CAD build for the part. Positions are in the model's coordinates, mm. A direction names the side the tool comes from. Give positions to 0.01 mm unless a question says otherwise; leave off trailing zeros. Loops run counter-clockwise (first coordinate to the right, second up) from the corner with the lowest first, then second, coordinate; pieces in that order, holes last. Notation, with made-up numbers: M 11,-20.75 L 35,-20.75 A28 ccw 35,3.25 Z; hole C 16.25,15 d8. An arc over 180 degrees is marked long. One line per question, with ' | ' between items.
```python
from build123d import *

# Parameters (mm, degrees)
F1_DEPTH  = 140
F3_DEPTH  = 25
F4_W      = 14.9999646693
F4_H      = 12.7701332697
F4_W_2    = 15
F5_DEPTH  = 2
F6_R      = 2
F7_W      = 11
F7_H      = 12
F8_DEPTH  = 2
F10_DEPTH = 50
F12_D     = 4.4


with BuildPart() as f1:
    # F0 (on Front) → F1 (new body)
    with BuildSketch(Plane.XZ):
        Polygon((-5.5, 12), (-7.5, 12), (-7.5, 0), (7.5, 0), (7.5, 12), (5.5, 12), (5.5, 2), (-5.5, 2), align=None)
    extrude(amount=F1_DEPTH)

    # F2 (on face) → F3 (cut)
    with BuildSketch(Plane(origin=(-7.5, 0, 0), x_dir=(0, -1, 0), z_dir=(-1, 0, 0))):
        Polygon((4.3676428112, 0), (0, 12), (0, 0), align=None)
    extrude(amount=-F3_DEPTH, mode=Mode.SUBTRACT)

    # F4 (on face) → F5 (join)
    with BuildSketch(Plane(origin=(0, -3.8567256581, 1.4037333413), x_dir=(-1, 0, 0), z_dir=(0, 0.9396926208, -0.3420201433))):
        with Locations((-12.9999823347, 4.8912448146)):
            Rectangle(F4_W, F4_H)
        with Locations((13, 4.8912448146)):
            Rectangle(F4_W_2, F4_H)
    extrude(amount=F5_DEPTH)

    # F6
    f6_edges = [f1.edges().sort_by_distance(p)[0] for p in [
        (20.499965, 0.939693, 11.65798),
        (-20.5, 0.939693, 11.65798),
        (20.499965, -3.42795, -0.34202),
        (-20.5, -3.42795, -0.34202),
    ]]
    fillet(f6_edges, radius=F6_R)

    # F7 (on face) → F8 (join)
    with BuildSketch(Plane(origin=(0, 0, 0), x_dir=(1, 0, 0), z_dir=(0, 0, -1))):
        with Locations((0, -1.6323571888)):
            Rectangle(F7_W, F7_H)
    extrude(amount=-F8_DEPTH)

    # F9 (on face) → F10 (cut, symmetric)
    with BuildSketch(Plane(origin=(-5.5, 0, 0), x_dir=(0, -1, 0), z_dir=(-1, 0, 0))):
        Polygon((2.2392872662, 0), (-7.6323571888, 0), (-7.6323571888, -1.849311986), (7.0655047894, -1.849311986), (7.0655047894, 0), align=None)
    extrude(amount=F10_DEPTH, both=True, mode=Mode.SUBTRACT)

    # F12 (through all)
    with Locations(Plane(origin=(0, -1.9773404165, 0.7196930546), x_dir=(-1, 0, 0), z_dir=(0, 0.9396926208, -0.3420201433))):
        with Locations((-12.5, 5.2763114494), (12.5, 5.2763114494)):
            Hole(F12_D / 2)


solid = f1.part
```
Item 1: Drill centre lines: line 1 along X through (y, z) = (-130.5, 11); line 2 along Z through (x, y) = (1, -122.5); line 3 along Y through (x, z) = (-17, 6.5). Where is each one in solid material? Low to high. Write a range as [from, to].
Conclusion:
line 1: [-7.5, -5.5], [5.5, 7.5] | line 2: [0, 2] | line 3: [-2, 0.13]
Item 2: Saw through at B-B on x = -13. Give the cut face in (y, z), and give its area (3 significant figures).
Conclusion:
outline: M -4.37,0 L -2.24,0 L -0.91,3.66 L -2.78,4.35 Z; M -1.32,8.38 L 0.56,7.69 L 1.88,11.32 L 0,12 Z | area: 16.2 mm²
Item 3: Saw through at A-A on y = -66.5. Give the cut face in (x, z), and give its area (3 significant figures).
Conclusion:
outline: M -7.5,0 L 7.5,0 L 7.5,12 L 5.5,12 L 5.5,2 L -5.5,2 L -5.5,12 L -7.5,12 Z | area: 70.0 mm²
Item 4: Saw through at C-C on x = -3.5. Give the cut face in (y, z).
Conclusion:
outline: M -140,0 L 7.63,0 L 7.63,2 L -140,2 Z
Item 5: Saw through at D-D on x = 17. Give the cut face in (y, z), and give its area (3 significant figures).
Conclusion:
outline: M -4.37,0 L -2.24,0 L 1.88,11.32 L 0,12 Z | area: 24.8 mm²
Item 6: 3-axis set-ups, long thin cutter, end or side, ignore diameter. For faces 1 (the flat face through (-15.353, -2.153, 6.084)), 2 (the flat face through (-14.6, -0.6, 4.5)), 3 (the flat face through (14.8, -0.6, 4.5)), 4 (the flat face through (0, -67, 2)): which of +Z, -Z, +X, -X, +Y, -Y reach the whole face in a straight line?
Conclusion:
face 1: +Z, -X, -Y | face 2: -Z, -X, +Y | face 3: -Z, +X, +Y | face 4: +Z, +Y, -Y
Item 7: Drop flat-ended pins along their axis: P1, Ø10, axis at x = 3, y = -106, coming from the -Z side; P2, Ø5, axis at y = -97.5, z = 9, coming from the -X side; P3, Ø3, axis at y = -45, z = 5.5, coming from the +X side; P4, Ø2, axis at y = 4.5, z = 0.5, coming from the -X side. Give the stop position or say it passes through.
Conclusion:
P1: z = 0 | P2: x = -7.5 | P3: x = 7.5 | P4: x = -5.5
Item 8: Mould opens along X. For faces 5 (the cylindrical face through (-10.47, -1.41, 5.23)), 6 (the flat face through (15.535, -2.153, 6.084)), 7 (the flat face through (5.5, -71, 7)), 8 (the flat face through (-20.5, -1, 6)) say: pulls with the +X half, pulls with the -X half, needs draft (parallel to the pull), parting line crosses it, or undercut.
Conclusion:
face 5: undercut | face 6: needs draft | face 7: undercut | face 8: pulls with the -X half
